Geometry check sheet. Reference: drawing and pictorial views, mm from the part's lowest x, y, z. Round coordinates to 2 decimals unless told otherwise and drop trailing zeros. Order: outer loops, then holes, each group sorted by start corner. A loop starts at its lowest first (then second) coordinate and runs counter-clockwise, first axis right, second up.
(1) Go/stop test with flat-tipped pins: pin 1 (4 mm diameter, centred on x = 4, z = 21.4, fed in from +Y); pin 2 (1.5 mm diameter, centred on x = 29.5, y = 1.5, fed in from -Z); pin 3 (2 mm diameter, centred on x = 39, y = 3, fed in from +Z). Record where each tip stops, or that it passes through.
(2) Material ranges on line 1 along X through (y, z) = (2.4, 21.4) (3 decimals); line 2 along Z through (x, y) = (56.5, 2.8) (1 decimal); line 3 along Z through (x, y) = (57.5, 0.55) (1 decimal), recorded low to high.
(3) Sectioned sample at B-B (z = 21.4). Record the boundary of the cut face in (x, y) (3 decimals).
(4) Sectioned sample at D-D (z = 35.5). Record the boundary of the cut face in (x, y).
(5) Sectioned sample at A-A (y = 2.5). Give the number of separate pieces and of enclosed holes in the cut face, plus the area to 3 significant figures.
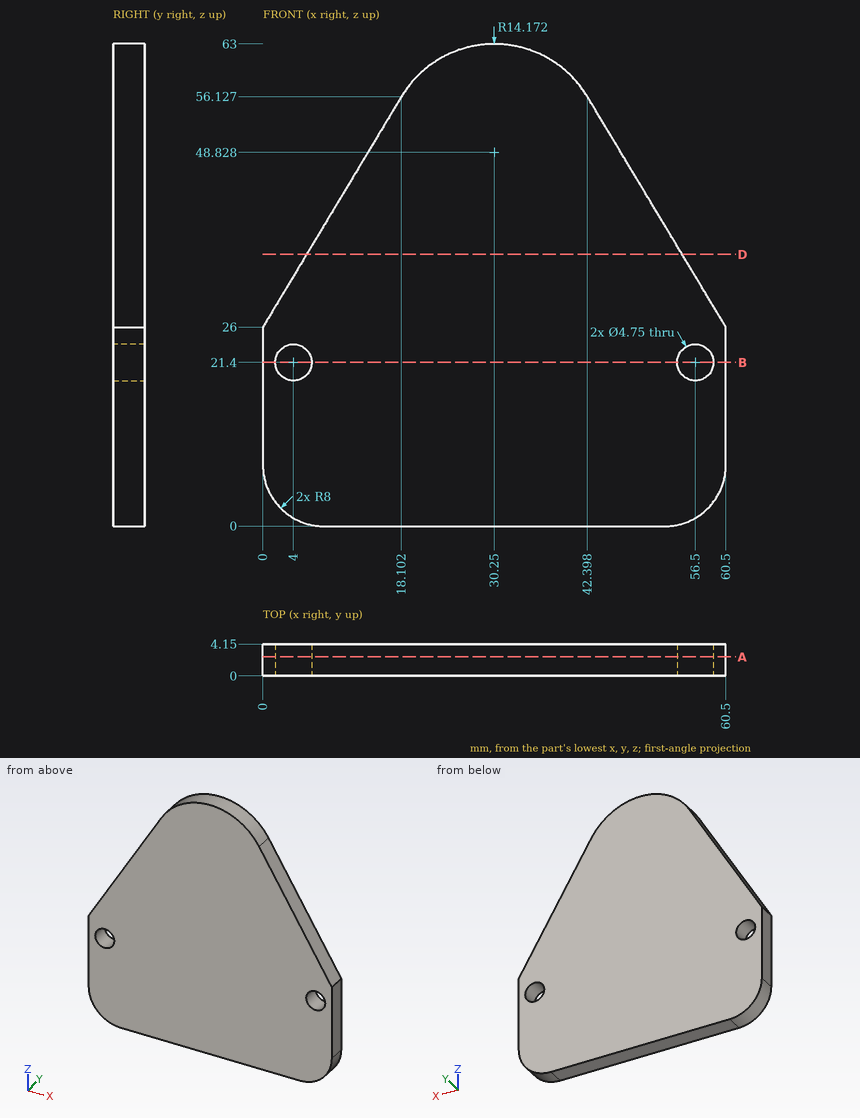
Answer below:
1. pin 1: passes through
1. pin 2: stops at z = 0
1. pin 3: stops at z = 60.69
2. line 1: x = 0 to 1.625, 6.375 to 54.125, 58.875 to 60.5
2. line 2: z = 1.1 to 19, 23.8 to 32.7
2. line 3: z = 1.8 to 19.2, 23.6 to 31
3. outline: (0, 0) - (1.625, 0) - (1.625, 4.15) - (0, 4.15) - close; (6.375, 0) - (54.125, 0) - (54.125, 4.15) - (6.375, 4.15) - close; (58.875, 0) - (60.5, 0) - (60.5, 4.15) - (58.875, 4.15) - close
4. outline: (5.71, 0) - (54.79, 0) - (54.79, 4.15) - (5.71, 4.15) - close
5. separate pieces: 1
5. enclosed holes: 2
5. area: 2,910 mm2
